Here's how the part is built. I have some questions about the finished solid (model axes, mm). Face numbers are marked on the shaded views. A direction names the side the tool comes from. Round coordinates to 2 decimals unless told otherwise and drop trailing zeros. Write each loop counter-clockwise with the first axis right and the second up, starting at its lowest first coordinate (ties: lowest second). Pieces come first, ordered by that corner, then holes. Notation, with made-up numbers: (77, -35.5) -> (83, -35.5) arc R27 ccw to (83, -7.5) -> close; hole circle Ø6 at (-5, 30.25). An arc over 180 degrees is marked (long way). Answer as CSV lines item,"result".
```python
from build123d import *

# Parameters (mm, degrees)
F0_W     = 25
F0_H     = 25
F0_W_2   = 5
F0_H_2   = 5
F1_DEPTH = 12.5
F2_W     = 25
F2_H     = 25
F3_DEPTH = 12.5


with BuildPart() as f1:
    # F0 (on Front) → F1 (new body)
    with BuildSketch(Plane.XZ):
        with Locations((12.5, 12.5)):
            Rectangle(F0_W, F0_H)
        Polygon((10, 16.5), (15, 16.5), (15, 11.5), (20, 11.5), (20, 6.5), (20, 1.5), (17.5, 1.5), (17.5, 6.5), (7.5, 6.5), (7.5, 1.5), (5, 1.5), (5, 6.5), (5, 11.5), (10, 11.5), align=None, mode=Mode.SUBTRACT)
        with Locations((7.5, 19.3)):
            Rectangle(F0_W_2, F0_H_2, mode=Mode.SUBTRACT)
        with Locations((17.5, 19.3)):
            Rectangle(F0_W_2, F0_H_2, mode=Mode.SUBTRACT)
    extrude(amount=F1_DEPTH)

    # F2 (on face) → F3 (join)
    with BuildSketch(Plane(origin=(0, 0, 0), x_dir=(-1, 0, 0), z_dir=(0, 1, 0))):
        with Locations((-12.5, 12.5)):
            Rectangle(F2_W, F2_H)
    extrude(amount=F3_DEPTH)


solid = f1.part
```
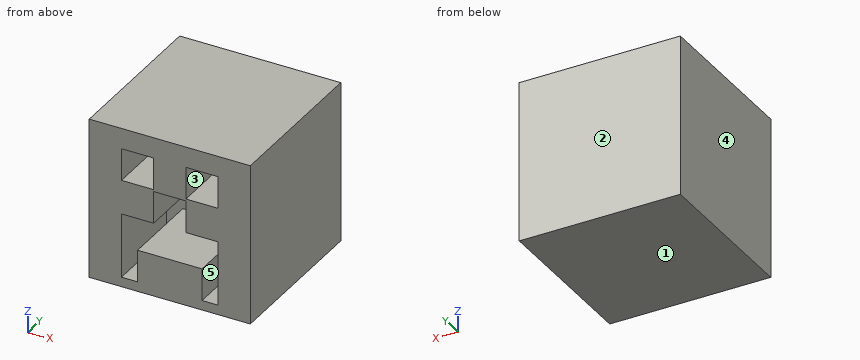
1. If we mould it in two halves opening along Z, with no side actions, what happens to the marked faces 1, 2 and 3? For each: released by +Z, released by -Z, zero draft, split by the parting line, or undercut.
Numbers:
face 1,"released by -Z"
face 2,"zero draft"
face 3,"undercut"
2. On a 3-axis mill with a long thin cutter (end or side, diameter ignored), from which of +Z, -Z, +X, -X, +Y, -Y can I reach the whole of each face in a straight line? I mean the marked faces 4 and 5. Say none if no direction works.
Numbers:
face 4,"+Z, -Z, -X, +Y, -Y"
face 5,"-Y"
3. For pin 1 Ø2.5 at (x, z) = (7, 20) entering from -Y, with a flat end and sliding along its axis, tell me the tip position at first contact or that it passes through.
Numbers:
pin 1,"stops at y = 0"
4. Suppose I cut it at B-B on y = -3.5. Please give me the cut outline in (x, z).
Numbers:
outline,"(0, 0) -> (25, 0) -> (25, 25) -> (0, 25) -> close; hole (5, 1.5) -> (7.5, 1.5) -> (7.5, 6.5) -> (17.5, 6.5) -> (17.5, 1.5) -> (20, 1.5) -> (20, 11.5) -> (15, 11.5) -> (15, 16.5) -> (10, 16.5) -> (10, 11.5) -> (5, 11.5) -> close; hole (5, 16.8) -> (10, 16.8) -> (10, 21.8) -> (5, 21.8) -> close; hole (15, 16.8) -> (20, 16.8) -> (20, 21.8) -> (15, 21.8) -> close"
5. If I drill on line 1 (Z direction, x = 7.25, y = -6.5); line 2 (X direction, y = -9.25, z = 3.5); line 3 (X direction, y = -1, z = 18.5), over which ranges is the centre line in solid material (lowest first)?
Numbers:
line 1,"z = 0 to 1.5, 11.5 to 16.8, 21.8 to 25"
line 2,"x = 0 to 5, 7.5 to 17.5, 20 to 25"
line 3,"x = 0 to 5, 10 to 15, 20 to 25"
6. Suppose I cut it at C-C on x = 11. Please give me the cut outline in (y, z), and give its area (3 significant figures).
Numbers:
outline,"(-12.5, 0) -> (12.5, 0) -> (12.5, 25) -> (-12.5, 25) -> (-12.5, 16.5) -> (0, 16.5) -> (0, 6.5) -> (-12.5, 6.5) -> close"
area,"500 mm^2"
7. Suppose I cut it at A-A on z = 5.25. Please give me the cut outline in (x, y), and give its area (4 significant figures).
Numbers:
outline,"(0, -12.5) -> (5, -12.5) -> (5, 0) -> (7.5, 0) -> (7.5, -12.5) -> (17.5, -12.5) -> (17.5, 0) -> (20, 0) -> (20, -12.5) -> (25, -12.5) -> (25, 12.5) -> (0, 12.5) -> close"
area,"562.5 mm^2"
8. Suppose I cut it at D-D on x = 5.5. Please give me the cut outline in (y, z).
Numbers:
outline,"(-12.5, 0) -> (12.5, 0) -> (12.5, 25) -> (-12.5, 25) -> (-12.5, 21.8) -> (0, 21.8) -> (0, 16.8) -> (-12.5, 16.8) -> (-12.5, 11.5) -> (0, 11.5) -> (0, 1.5) -> (-12.5, 1.5) -> close"
